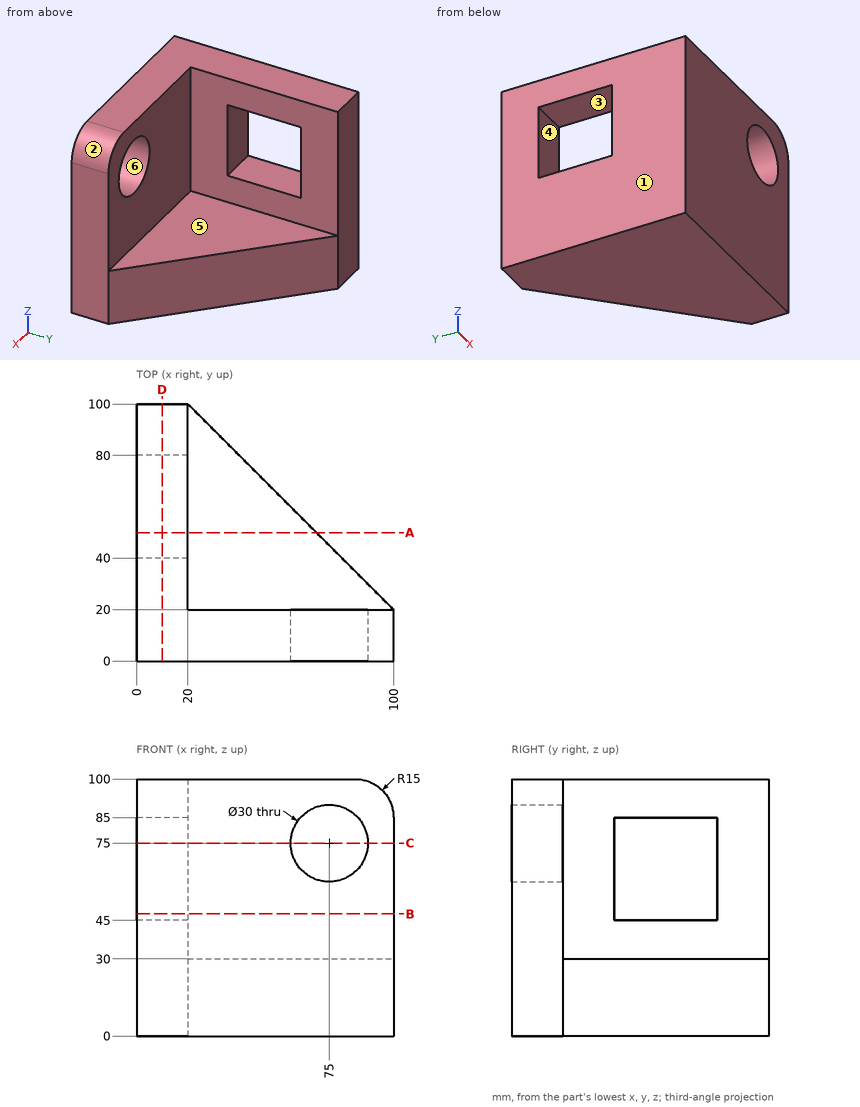
Geometry check sheet. Reference: drawing and pictorial views, mm from the part's lowest x, y, z. A direction names the side the tool comes from. Round coordinates to 2 decimals unless told otherwise and drop trailing zeros. Write each loop counter-clockwise with the first axis right and the second up, starting at its lowest first coordinate (ties: lowest second). Pieces come first, ordered by that corner, then holes.
(1) Section check A-A (y = 50). Enter the section's corners in (x, z), plus the area to 3 significant figures.
Returned:
outline: (0, 0) - (70, 0) - (70, 30) - (20, 30) - (20, 45) - (0, 45) - close; (0, 85) - (20, 85) - (20, 100) - (0, 100) - close
area: 2,700 mm2
(2) Material ranges on line 1 (Z direction, x = 75, y = 11); line 2 (Y direction, x = 88, z = 39), recorded low to high.
Returned:
line 1: z = 0 to 60, 90 to 100
line 2: y = 0 to 20
(3) Section check C-C (z = 75). Enter the section's corners in (x, y), plus the area to 3 significant figures.
Returned:
outline: (0, 0) - (60, 0) - (60, 20) - (20, 20) - (20, 40) - (0, 40) - close; (0, 80) - (20, 80) - (20, 100) - (0, 100) - close; (90, 0) - (100, 0) - (100, 20) - (90, 20) - close
area: 2,200 mm2
(4) Mould release check, pull along Z, two halves, no side actions. Record for the marked faces 1, 2 and 3: pulls with the +Z half, pulls with the -Z half, needs draft (parallel to the pull), parting line crosses it, or undercut.
Returned:
face 1: needs draft
face 2: pulls with the +Z half
face 3: undercut
(5) Section check D-D (x = 10). Enter the section's corners in (y, z), plus the area to 3 significant figures.
Returned:
outline: (0, 0) - (100, 0) - (100, 100) - (0, 100) - close; hole (40, 45) - (80, 45) - (80, 85) - (40, 85) - close
area: 8,400 mm2
(6) Depth check by flat-ended pin: pin 1 Ø24 at (x, y) = (54.5, 65.5) entering from +Z; pin 2 Ø12 at (x, y) = (76, 54.5) entering from +Z; pin 3 Ø21 at (y, z) = (74, 63) entering from +X; pin 4 Ø1.5 at (y, z) = (22.5, 29) entering from +X. Enter the tip coordinate at first touch or a pass-through.
Returned:
pin 1: stops at z = 30
pin 2: passes through
pin 3: stops at x = 20
pin 4: stops at x = 98.25
(7) Section check B-B (z = 47.5). Enter the section's corners in (x, y).
Returned:
outline: (0, 0) - (100, 0) - (100, 20) - (20, 20) - (20, 40) - (0, 40) - close; (0, 80) - (20, 80) - (20, 100) - (0, 100) - close
(8) Access from +Z, -Z, +X, -X, +Y, -Y to the whole of each face (thin tool, end or side, straight path). Record for the marked faces 4, 5 and 6.
Returned:
face 4: +X, -X
face 5: +Z, +X, +Y
face 6: +Y, -Y
